For this review, take the finished solid that the model builds, in its own axes (mm). Face numbers are marked on the shaded views. A direction names the side the tool comes from. Round coordinates to 2 decimals unless told otherwise and drop trailing zeros. Write each loop counter-clockwise with the first axis right and the second up, starting at its lowest first coordinate (ties: lowest second). Pieces come first, ordered by that corner, then holes. Notation, with made-up numbers: (68.5, 45) -> (116.5, 45) arc R29 ccw to (116.5, 69) -> close; hole circle Ø11 at (-37.5, 34). An arc over 180 degrees is marked (long way). Answer as CSV lines item,"result". Start each with the question number.
Item 1: Mouldability with a two-part tool opening along Y and no side actions: class the marked faces 1, 2 and 3 as +Y half, -Y half, draft (parallel to the pull), parting line (faces both ways), or undercut.
Item 2: Machinability: for the marked faces 4, 5 and 6, which of the approach directions +Z, -Z, +X, -X, +Y, -Y give a long, thin tool a straight path to every point of the face, cutting with its end or side? Answer none if there is none.
Item 3: Take a section at A-A on y = -5. Give the boundary of the cut face in (x, z).
Item 4: Wall thickness on probe 1 along Y at (x, z) = (30, 8.5); probe 2 along Y at (x, z) = (-1.5, 9); probe 3 along X at (y, z) = (-4, 10.75): over which ranges is each line inside the solid? List them lowest first. Write a range as from..to.
Item 5: Take a section at D-D on y = -11.5. Give the boundary of the cut face in (x, z).
Item 6: Take a section at B-B on x = 30. Give the boundary of the cut face in (y, z), then the cut area to 3 significant figures.
Item 7: For pin 1 Ø3.5 at (y, z) = (1, 8) entering from -X; pin 2 Ø3 at (x, z) = (37.5, 7) entering from -Y; pin 3 Ø2 at (x, z) = (37, 8) entering from +Y, all flat-tipped, find the tip position at first contact; note any pin that passes through.
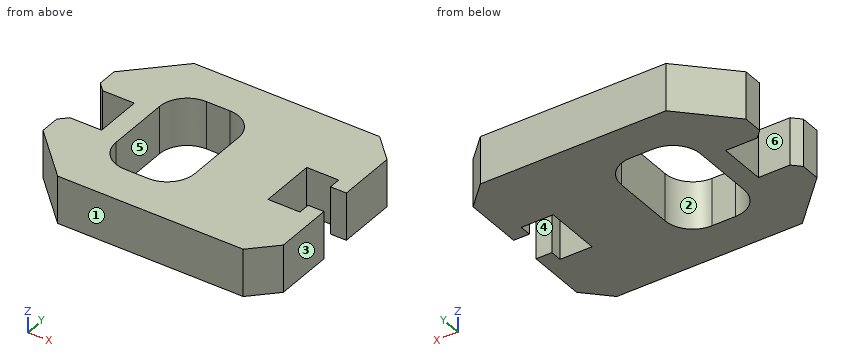
```python
from build123d import *

# Parameters (mm, degrees)
F1_DEPTH = 12
F2_W     = 12
F2_H     = 12
F3_DEPTH = 25
F4_SIZE  = 6
F5_W     = 20
F5_H     = 30
F6_DEPTH = 30
F7_R     = 7
F9_DEPTH = 25
F10_SIZE = 12
F11_SIZE = 2


with BuildPart() as f1:
    # F0 (on Top) → F1 (new body)
    with BuildSketch(Plane.XY):
        Polygon((40, 25), (-40, 25), (-40, -25), (40, -25), (40, -4.1), (36, -4.1), (36, -7.1), (27.9, -7.1), (27.9, 7.1), (36, 7.1), (36, 4.1), (40, 4.1), align=None)
    extrude(amount=F1_DEPTH)

    # F2 (on face) → F3 (cut)
    with BuildSketch(Plane(origin=(-40, 0, 0), x_dir=(0, -1, 0), z_dir=(-1, 0, 0))):
        with Locations((0, 6)):
            Rectangle(F2_W, F2_H)
    extrude(amount=-F3_DEPTH, mode=Mode.SUBTRACT)

    # F4
    f4_edges = [f1.edges().sort_by_distance(p)[0] for p in [
        (-40, -25, 6),
        (-40, 25, 6),
        (-40, 6, 6),
        (-40, -6, 6),
        (40, -25, 6),
        (40, 25, 6),
    ]]
    chamfer(f4_edges, length=F4_SIZE)

    # F5 (on face) → F6 (cut)
    with BuildSketch(Plane(origin=(0, 0, 0), x_dir=(1, 0, 0), z_dir=(0, 0, -1))):
        Rectangle(F5_W, F5_H)
    extrude(amount=-F6_DEPTH, mode=Mode.SUBTRACT)

    # F7
    f7_edges = [f1.edges().sort_by_distance(p)[0] for p in [
        (10, 15, 6),
        (-10, 15, 6),
        (-10, -15, 6),
        (10, -15, 6),
    ]]
    fillet(f7_edges, radius=F7_R)

    # F8 (on face) → F9 (cut)
    with BuildSketch(Plane(origin=(0, 0, 0), x_dir=(1, 0, 0), z_dir=(0, 0, -1))):
        Polygon((-41.9909754243, -28.1055098634), (-25, -28.1055098634), (-25, -25), (-34, -25), (-40, -19), (-40, -12), (-34, -6), (-25, -6), (-25, 6), (-34, 6), (-40, 12), (-40, 19), (-34, 25), (-25, 25), (-25, 27.3810768734), (-41.9909754243, 27.3810768734), align=None)
        Polygon((-34, -25), (-25, -25), (-25, -6), (-34, -6), (-40, -12), (-40, -19), align=None)
        Polygon((-34, 6), (-25, 6), (-25, 25), (-34, 25), (-40, 19), (-40, 12), align=None)
    extrude(amount=-F9_DEPTH, mode=Mode.SUBTRACT)

    # F10
    f10_edges = [f1.edges().sort_by_distance(p)[0] for p in [
        (-25, 25, 6),
        (-25, -25, 6),
    ]]
    chamfer(f10_edges, length=F10_SIZE)

    # F11
    f11_edges = [f1.edges().sort_by_distance(p)[0] for p in [
        (-25, 6, 6),
        (-25, -6, 6),
    ]]
    chamfer(f11_edges, length=F11_SIZE)


solid = f1.part
```
Output values:
1,face 1,"-Y half"
1,face 2,"undercut"
1,face 3,"draft"
2,face 4,"+Z, -Z, +X"
2,face 5,"+Z, -Z"
2,face 6,"+Z, -Z, -X"
3,outline,"(-15, 0) -> (-10, 0) -> (-10, 12) -> (-15, 12) -> close; (10, 0) -> (27.9, 0) -> (27.9, 12) -> (10, 12) -> close; (36, 0) -> (40, 0) -> (40, 12) -> (36, 12) -> close"
4,probe 1,"y = -25..-7.1, 7.1..25"
4,probe 2,"y = -25..-15, 15..25"
4,probe 3,"x = -15..-10, 10..27.9"
5,outline,"(-25, 0) -> (-9.06, 0) -> (-9.06, 12) -> (-25, 12) -> close; (9.06, 0) -> (40, 0) -> (40, 12) -> (9.06, 12) -> close"
6,outline,"(-25, 0) -> (-7.1, 0) -> (-7.1, 12) -> (-25, 12) -> close; (7.1, 0) -> (25, 0) -> (25, 12) -> (7.1, 12) -> close"
6,area,"430 mm^2"
7,pin 1,"stops at x = -15"
7,pin 2,"stops at y = -23"
7,pin 3,"stops at y = 23"
